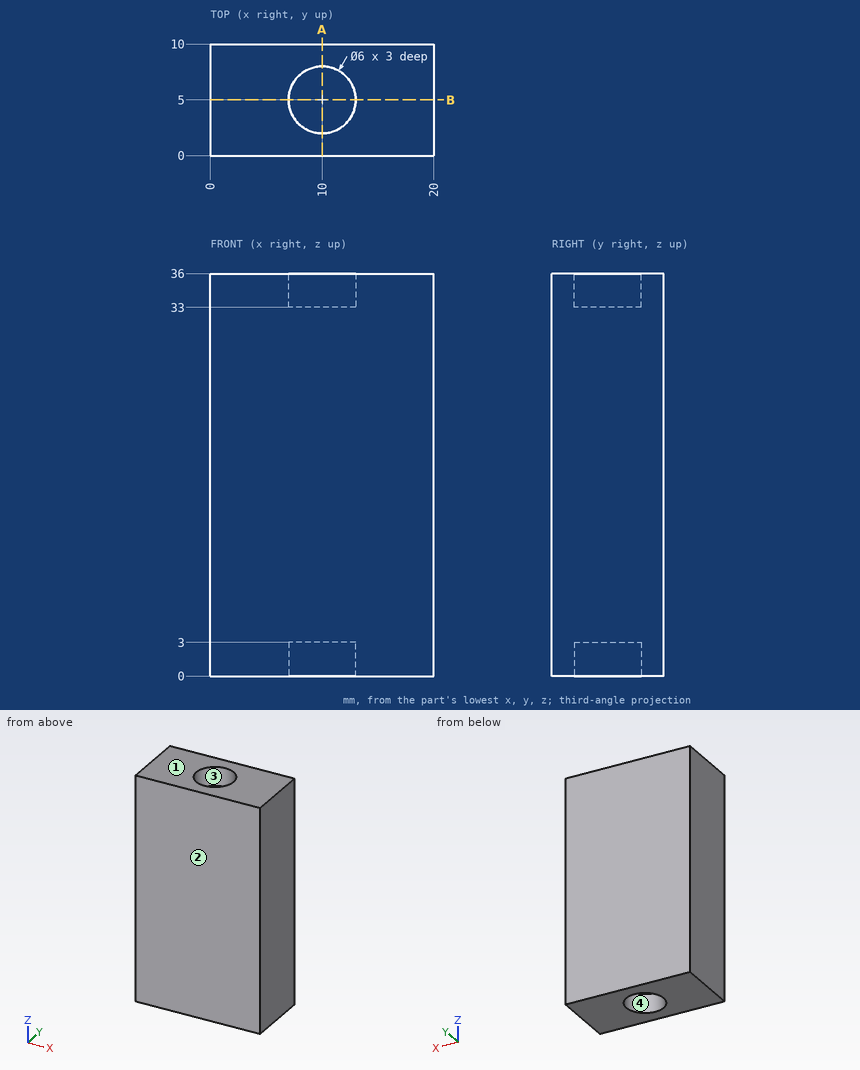
The drawing under review shows one solid part. Ordinate dimensions are in mm from its lowest x, y, z. Coordinates: 2 decimals unless noted, no trailing zeros. Write each loop counter-clockwise with the first axis right and the second up, starting at its lowest first coordinate (ties: lowest second). Pieces come first, ordered by that corner, then holes. Notation, with made-up numbers: (16.25, -40) -> (61.25, -40) arc R18 cw to (61.25, -28) -> close; hole circle Ø6 at (33, 69.5). An arc over 180 degrees is marked (long way). Write each question's results on one line, items separated by ' | '. Start each with the question number.
1) The part is to be moulded in two halves that separate along Y. For the marked faces 1, 2, 3 and 4, say which applies: +Y half, -Y half, draft (parallel to the pull), parting line (faces both ways), or undercut.
2) Wall thickness on L1, parallel to X at y = 5, z = 2; L2, parallel to Y at x = 10, z = 1.5; L3, parallel to Z at x = 10.25, y = 4.25: over which ranges is each line inside the solid? List them lowest first. Write a range as [from, to].
3) Insertion check: pin 1 (5 mm diameter, centred on x = 10, y = 5, fed in from +Z); pin 2 (3 mm diameter, centred on x = 10.5, y = 4, fed in from -Z). Each pin has a flat end and moves straight along its axis. Give the tip position at first contact, or say it passes through.
4) Consider section B-B (y = 5). Write out the cut boundary in (x, z), plus the area to 3 significant figures.
5) Consider section A-A (x = 10). Write out the cut boundary in (y, z), plus the area to 3 significant figures.
Geometry says:
1) face 1: draft | face 2: -Y half | face 3: undercut | face 4: undercut
2) L1: [0, 7], [13, 20] | L2: [0, 2], [8, 10] | L3: [3, 33]
3) pin 1: z = 33 | pin 2: z = 3
4) outline: (0, 0) -> (7, 0) -> (7, 3) -> (13, 3) -> (13, 0) -> (20, 0) -> (20, 36) -> (13, 36) -> (13, 33) -> (7, 33) -> (7, 36) -> (0, 36) -> close | area: 684 mm^2
5) outline: (0, 0) -> (2, 0) -> (2, 3) -> (8, 3) -> (8, 0) -> (10, 0) -> (10, 36) -> (8, 36) -> (8, 33) -> (2, 33) -> (2, 36) -> (0, 36) -> close | area: 324 mm^2
